Autodesk Inventor part; units mm, degrees
ref_plane "YZ Plane" through (0, 0, 0) normal (1, 0, 0) x (0, 1, 0)
ref_plane "XZ Plane" through (0, 0, 0) normal (0, 1, 0) x (-1, 0, 0)
ref_plane "XY Plane" through (0, 0, 0) normal (0, 0, 1) x (1, 0, 0)
sketch "Sketch1" plane through (0, 0, 0) normal (0, 1, 0) x (-1, 0, 0)
  line L0 (15.875, 31.75) -> (-15.875, 31.75)
  line L1 (-15.875, 31.75) -> (-15.875, -31.75)
  line L2 (-15.875, -31.75) -> (15.875, -31.75)
  line L3 (15.875, -31.75) -> (15.875, 31.75)
  line L4 (15.875, 31.75) -> (-15.875, -31.75) construction
  line L5 (-15.875, 31.75) -> (15.875, -31.75) construction
  line L6 (12.7, 28.575) -> (-12.7, 28.575)
  line L7 (-12.7, 28.575) -> (-12.7, -28.575)
  line L8 (-12.7, -28.575) -> (12.7, -28.575)
  line L9 (12.7, -28.575) -> (12.7, 28.575)
  line L10 (12.7, 28.575) -> (-12.7, -28.575) construction
  line L11 (-12.7, 28.575) -> (12.7, -28.575) construction
  point P0 (0, 0)
  dimension "d0" = 63.5
  dimension "d1" = 3.175
  dimension "d26" = 3.175
  dimension "d27" = 31.75
extrude "Extrusion1" add sketch "Sketch1" along normal blind 1143
sketch "Sketch4" plane through (-15.875, 0, 31.75) normal (0, 0, 1) x (1, 0, 0)
  line L0 (15.875, 0) -> (15.875, 1143) construction
  line L1 (15.875, 304.8) -> (15.875, 1041.4) construction
  line L2 (19.05, 304.8) -> (19.05, 1041.4)
  line L3 (12.7, 1041.4) -> (12.7, 304.8)
  arc A0 (12.7, 304.8) -> (19.05, 304.8) centre (15.875, 304.8) ccw
  arc A1 (19.05, 1041.4) -> (12.7, 1041.4) centre (15.875, 1041.4) ccw
  line L4 (0, 1143) -> (31.75, 1143)
  line L5 (0, 0) -> (31.75, 0)
  point P0 (15.875, 673.1)
  dimension "d6" = 6.35
  dimension "d7" = 101.6
  dimension "d8" = 304.8
  dimension "d28" = 736.6
extrude "Extrusion3" cut sketch "Sketch4" against normal through all
sketch "Sketch5" plane through (15.875, 0, 31.75) normal (1, 0, 0) x (0, 0, -1)
  circle A0 centre (31.75, 127) radius 4.7625
  line L0 (0, 0) -> (63.5, 0)
  line L1 (0, 0) -> (0, 1143)
  point P0 (31.75, 0)
  dimension "d11" = 9.525
  dimension "d12" = 127
  dimension "d25" = 31.75
extrude "Extrusion4" cut sketch "Sketch5" against normal up to next
sketch "Sketch6" plane through (-15.875, 0, 31.75) normal (0, 0, 1) x (1, 0, 0)
  circle A0 centre (15.875, 50.8) radius 4.7625
  line L0 (0, 0) -> (31.75, 0)
  line L1 (0, 0) -> (0, 1143)
  point P0 (15.875, 0)
  dimension "d15" = 9.525
  dimension "d16" = 50.8
  dimension "d24" = 15.875
extrude "Extrusion5" cut sketch "Sketch6" against normal through all
sketch "Sketch7" plane through (15.875, 0, 31.75) normal (1, 0, 0) x (0, 0, -1)
  circle A0 centre (31.75, 50.8) radius 4.7625
  line L0 (0, 0) -> (63.5, 0)
  line L1 (31.75, 0) -> (31.75, 96.4703) construction
  line L2 (0, 0) -> (0, 1143) construction
  dimension "d19" = 9.525
  dimension "d20" = 50.8
  dimension "d23" = 31.75
extrude "Extrusion6" cut sketch "Sketch7" against normal through all
sketch "Sketch8" plane through (15.875, 0, 31.75) normal (1, 0, 0) x (0, 0, -1)
  circle A0 centre (25.4, 330.2) radius 4.7625
  line L0 (0, 1143) -> (63.5, 1143)
  point P0 (31.75, 0)
  dimension "d29" = 9.525
  dimension "d30" = 812.8
extrude "Extrusion7" cut sketch "Sketch8" against normal through all
equation "\"d0\" = tubeBreadth"
equation "\"d1\" = tubeThickness"
equation "\"d27\" = tubeWidth"
equation "\"d2\" = tubeLength"
equation "\"d6\" = slotWidth"
equation "\"d7\" = slotDistanceFromTop"
equation "\"d8\" = slotDistanceFromBottom"
equation "\"d25\" = 0.5 * tubeBreadth"
equation "\"d15\" = axelDiam"
equation "\"d16\" = axelHeightAboveBottomOfTube"
equation "\"d24\" = 0.5 * tubeWidth"
equation "\"d19\" = axelDiam"
equation "\"d20\" = axelHeightAboveBottomOfTube"
equation "\"d23\" = 0.5 * tubeBreadth"
equation "\"d29\" = stopHoleDiam"
equation "\"d30\" = stopHoleDistanceFromTop"
equation "\"tubeBreadth\" = 63.5"
equation "\"tubeThickness\" = 3.175"
equation "\"tubeLength\" = 1143"
equation "\"slotDistanceFromBottom\" = 304.8"
equation "\"slotDistanceFromTop\" = 101.6"
equation "\"slotWidth\" = 6.35"
equation "\"axelDiam\" = 9.525"
equation "\"axelHeightAboveBottomOfTube\" = 50.8"
equation "\"tubeWidth\" = 31.75"
equation "\"stopHoleDiam\" = 9.525"
properties part number "OuterTube" material "Aluminum 6061"
Read the model definition and answer for the solid it produces. Units are mm, in the model's axes. A direction names the side the tool comes from. Coordinates: 2 decimals unless noted, no trailing zeros. Loops run counter-clockwise (first coordinate to the right, second up) from the corner with the lowest first, then second, coordinate; pieces in that order, holes last. Notation, with made-up numbers: (88.5, 66.25) -> (93.5, 66.25) arc R24 cw to (93.5, 83.25) -> close; hole circle Ø6 at (-12.5, 49). An arc over 180 degrees is marked (long way). Write item = value, one per line. Start each with the question number.
1) The mould has two halves that part along X. Classify faces 3 (the face through (13, 0, 3)), 4 (the face through (-12.7, 563, 0)), 5 (the face through (15.875, 563, 0)): pulls with the +X half, pulls with the -X half, needs draft (parallel to the pull), parting line crosses it, or undercut.
2) Given P1, Ø12.5, axis at y = 330.2, z = 6.35, coming from the -X side (3 decimals); P2, Ø10, axis at x = -1, z = -20, coming from the -Y side, each flat-ended and moving along its own axis, determine where each tip first touches the part or whether it passes through.
3) Find the intervals of material crossed by L1, parallel to Y at x = 0, z = 29.6 (1 decimal); L2, parallel to X at y = 707, z = 0.5 (3 decimals); L3, parallel to Z at x = 5, y = 304 (3 decimals), in increasing order. Write a range as from..to.
4) The part is cut by section A-A, the plane y = 702. Determine the outline of the cut face in (x, z) (3 decimals).
5) For faces 1 (the face through (-15.875, 563, 0)), 2 (the face through (5, 563, 28.575)), determine the directions among +Z, -Z, +X, -X, +Y, -Y from which every point of the face is accessible in a straight line to the end or side of a thin tool.
Result:
q1.face_3 = needs draft
q1.face_4 = undercut
q1.face_5 = pulls with the +X half
q2.P1 = -15.875
q2.P2 = through
q3.L1 = 0..46, 55.6..301.6, 1044.6..1143
q3.L2 = -15.875..-12.7, 12.7..15.875
q3.L3 = -31.75..-28.575, 28.575..31.75
q4.outline = (-15.875, -31.75) -> (-3.175, -31.75) -> (-3.175, -28.575) -> (-12.7, -28.575) -> (-12.7, 28.575) -> (-3.175, 28.575) -> (-3.175, 31.75) -> (-15.875, 31.75) -> close; (3.175, -31.75) -> (15.875, -31.75) -> (15.875, 31.75) -> (3.175, 31.75) -> (3.175, 28.575) -> (12.7, 28.575) -> (12.7, -28.575) -> (3.175, -28.575) -> close
q5.face_1 = +Z, -Z, -X, +Y, -Y
q5.face_2 = +Y, -Y
